The listing builds one solid part. Answer for the finished solid, in the listing's coordinates (mm). A direction names the side the tool comes from. Coordinates: 2 decimals unless noted, no trailing zeros. Loops run counter-clockwise (first coordinate to the right, second up) from the corner with the lowest first, then second, coordinate; pieces in that order, holes last. Notation, with made-up numbers: M 56,-5 L 92,-5 A26 ccw 92,20 Z; hole C 77,49 d5. An arc over 180 degrees is marked long. Return JSON: item names as keys, results as strings. Group by question number.
1. Section C-C (y = -0.75) is taken. Write down the section's boundary in (x, z), then the cut area to 3 significant figures.
2. Section B-B (z = 18) is taken. Write down the section's boundary in (x, y).
3. Section A-A (y = -4.5) is taken. Write down the section's boundary in (x, z).
4. Given P1, Ø1, axis at y = -5, z = -11, coming from the -X side; P2, Ø1, axis at x = 11, y = -6, coming from the -Z side; P3, Ø3, axis at x = -3, z = 2, coming from the +Y side; P4, Ø5, axis at x = -8.5, y = -7, coming from the -Z side, each flat-ended and moving along its own axis, determine where each tip first touches the part or whether it passes through.
5. Which of the six approach directions +Z, -Z, +X, -X, +Y, -Y give full straight-line access (tool end or side, diameter ignored) to faces 4 (the face through (-5, -13, -5)), 5 (the face through (11, -2, 10)), 6 (the face through (10, -6, 0.5)), 7 (the face through (13, -9, -2))?
6. Section D-D (z = 0) is taken. Write down the section's boundary in (x, y).
7. Straight lines are drawn through the part: L1, parallel to Z at x = 0, y = -4.75; L2, parallel to Z at x = 9.5, y = -7.5; L3, parallel to Z at x = 0.5, y = -6.5. For each, find the intervals that lie inside material, in ascending order. Write a range as from..to.
8. The mould has two halves that part along X. Classify faces 1 (the face through (7.04, -4.44, 15.06)), 2 (the face through (10, -4.43, 5.06)), 3 (the face through (0.36, -4.44, 23.49)): pulls with the +X half, pulls with the -X half, needs draft (parallel to the pull), parting line crosses it, or undercut.
```python
from build123d import *

# Parameters (mm, degrees)
SKETCH001_W     = 13
SKETCH001_H     = 6.5
SKETCH_R        = 2.5
SKETCH_R_2      = 10
PAD_DEPTH       = 9
SKETCH002_R     = 1.5
POCKET_DEPTH    = 33.501
CHAMFER_SIZE    = 0.75
CHAMFER001_SIZE = 0.5
FILLET_R        = 0.5
SKETCH003_W     = 16
SKETCH003_H     = 1
POCKET001_DEPTH = 13.001


with BuildPart() as shaft_support:
    # Sketch001 → Revolution (revolve)
    with BuildSketch(Plane.YZ):
        with Locations((-6.5, 9.25)):
            Rectangle(SKETCH001_W, SKETCH001_H)
    revolve(axis=Axis((0, 0, 0), (0, 1, 0)))


with BuildPart() as obj1:
    # Sketch → Pad (new body)
    with BuildSketch(Plane.XZ):
        with BuildLine():
            Line((-14, -2.5), (-14, 2.5))
            Line((-14, 2.5), (-4.908286, 20.481678))
            ThreePointArc((5.128166, 19.987941), (0.270242, 23.493357), (-4.908286, 20.481678))
            Line((5.128166, 19.987941), (9, 10))
            Line((9, 10), (14, 10))
            Line((14, 10), (14, -10))
            Line((14, -10), (9, -10))
            Line((9, -10), (5.128167, -19.987938))
            ThreePointArc((-4.908296, -20.481659), (0.270233, -23.493357), (5.128167, -19.987938))
            Line((-4.908296, -20.481659), (-14, -2.5))
        make_face()
        with Locations((0, 18)):
            Circle(SKETCH_R, mode=Mode.SUBTRACT)
        with Locations((0, -18)):
            Circle(SKETCH_R, mode=Mode.SUBTRACT)
        Circle(SKETCH_R_2, mode=Mode.SUBTRACT)
    extrude(amount=PAD_DEPTH)

    # Fusion: union shaft-support
    add(shaft_support.part)

    # Sketch002 → Pocket (cut, through all)
    with BuildSketch(Plane.XY.offset(10)):
        with Locations((11.5, -4.5)):
            Circle(SKETCH002_R)
    extrude(amount=-POCKET_DEPTH, mode=Mode.SUBTRACT)

    # Chamfer
    chamfer_edges = [obj1.edges().sort_by_distance(p)[0] for p in [
        (0, -13, -6),
    ]]
    chamfer(chamfer_edges, length=CHAMFER_SIZE)

    # Chamfer001
    chamfer001_edges = [obj1.edges().sort_by_distance(p)[0] for p in [
        (10, -4.5, 10),
        (10, -4.5, -10),
    ]]
    chamfer(chamfer001_edges, length=CHAMFER001_SIZE)

    # Fillet
    fillet_edges = [obj1.edges().sort_by_distance(p)[0] for p in [
        (0, -13, -12.5),
    ]]
    fillet(fillet_edges, radius=FILLET_R)

    # Sketch003 → Pocket001 (cut, through all)
    with BuildSketch(Plane(origin=(0, 0, 0), x_dir=(-1, 0, 0), z_dir=(0, 1, 0))):
        with Locations((-8, 0)):
            Rectangle(SKETCH003_W, SKETCH003_H)
    extrude(amount=-POCKET001_DEPTH, mode=Mode.SUBTRACT)


solid = obj1.part
```
Worked out:
{
 "1": {"outline": "M -14,-2.5 L -4.91,-20.48 A5.5 ccw 5.13,-19.99 L 9,-10 L 14,-10 L 14,-0.5 L 5.98,-0.5 A6 cw long 5.98,0.5 L 14,0.5 L 14,10 L 9,10 L 5.13,19.99 A5.5 ccw -4.91,20.48 L -14,2.5 Z; hole C 0,-18 d5; hole C 0,18 d5", "area": "718 mm^2"},
 "2": {"outline": "M -6.16,-9 L -2.5,-9 L -2.5,0 L -6.16,0 Z; M 2.5,-9 L 5.9,-9 L 5.9,0 L 2.5,0 Z"},
 "3": {"outline": "M -14,-2.5 L -4.91,-20.48 A5.5 ccw 5.13,-19.99 L 9,-10 L 9.5,-10 L 10,-9.5 L 10,-0.5 L 5.98,-0.5 A6 cw long 5.98,0.5 L 10,0.5 L 10,9.5 L 9.5,10 L 9,10 L 5.13,19.99 A5.5 ccw -4.91,20.48 L -14,2.5 Z; M 13,-9.5 L 13.5,-10 L 14,-10 L 14,-0.5 L 13,-0.5 Z; M 13,0.5 L 14,0.5 L 14,10 L 13.5,10 L 13,9.5 Z; hole C 0,-18 d5; hole C 0,18 d5"},
 "4": {"P1": "x = -9.96", "P2": "z = -10", "P3": "through", "P4": "z = -18.32"},
 "5": {"face 4": "+Z, -Z, +X, -X, -Y", "face 5": "+Z, +X, +Y, -Y", "face 6": "+X, +Y, -Y", "face 7": "-Y"},
 "6": {"outline": "M -14,-9 L -12.5,-9 L -12.5,-12.5 A0.5 ccw -12,-13 L -6.75,-13 L -6,-12.25 L -6,0 L -14,0 Z"},
 "7": {"L1": "-23.5..-20.5, -15.5..-6, 6..15.5, 20.5..23.5", "L2": "-10..-0.5, 0.5..10", "L3": "-23.48..-20.45, -15.55..-5.98, 5.98..15.55, 20.45..23.48"},
 "8": {"face 1": "pulls with the +X half", "face 2": "undercut", "face 3": "parting line crosses it"}
}
